```python
from build123d import *

# Parameters (mm, degrees)
SKETCH_1_W          = 106.8
SKETCH_1_H          = 58.8
EXTRUDE_1_DEPTH     = 8
CUT_EXTRUDE_1_DEPTH = 6.08
EXTRUDE_START       = 2.5
EXTRUDE_2_DEPTH     = 2.5
SKETCH_4_W          = 27.87
SKETCH_4_H          = 2.8
CUT_EXTRUDE_2_DEPTH = 4
EXTRUDE_START_2     = 4.5
EXTRUDE_3_DEPTH     = 4.5
SKETCH_6_R          = 1.9
CUT_EXTRUDE_3_DEPTH = 38.5
SKETCH_7_R          = 3.25
CUT_EXTRUDE_4_DEPTH = 3
CHAMFER_7_SIZE      = 0.5
CUT_EXTRUDE_5_DEPTH = 3
CHAMFER_6_SIZE      = 0.5
EXTRUDE_4_DEPTH     = 3
CUT_EXTRUDE_6_DEPTH = 3


with BuildPart() as part:
    # Sketch 1 → Extrude 1 (new body)
    with BuildSketch(Plane(origin=(0, 0, 0), x_dir=(1, 0, 0), z_dir=(0, 1, 0))):
        Rectangle(SKETCH_1_W, SKETCH_1_H)
    extrude(amount=EXTRUDE_1_DEPTH)

    # Sketch 2 → Cut-Extrude 1 (cut)
    with BuildSketch(Plane(origin=(0, 8, 0), x_dir=(1, 0, 0), z_dir=(0, 1, 0))):
        with BuildLine():
            Line((-46.75, -21.5), (46.75, -21.5))
            ThreePointArc((46.75, -21.5), (50.285533906, -20.035533906), (51.75, -16.5))
            Line((51.75, -16.5), (51.75, 24.6))
            ThreePointArc((51.75, 24.6), (51.164213562, 26.014213562), (49.75, 26.6))
            Line((49.75, 26.6), (21.23, 26.6))
            ThreePointArc((21.23, 26.6), (19.815786438, 26.014213562), (19.23, 24.6))
            Line((19.23, 24.6), (19.23, 23.05))
            ThreePointArc((19.23, 23.05), (18.644213562, 21.635786438), (17.23, 21.05))
            Line((17.23, 21.05), (-46.75, 21.05))
            ThreePointArc((-46.75, 21.05), (-50.285533906, 19.585533906), (-51.75, 16.05))
            Line((-51.75, 16.05), (-51.75, -16.5))
            ThreePointArc((-51.75, -16.5), (-50.285533906, -20.035533906), (-46.75, -21.5))
        make_face()
    extrude(amount=-CUT_EXTRUDE_1_DEPTH, mode=Mode.SUBTRACT)

    # Sketch 3 → Extrude 2 (add)
    with BuildSketch(Plane(origin=(0, 8, 0), x_dir=(1, 0, 0), z_dir=(0, 1, 0)).offset(EXTRUDE_START)):
        with BuildLine():
            Line((51.75, 21.1), (53.4, 21.1))
            Line((53.4, 21.1), (53.4, 29.4))
            Line((53.4, 29.4), (49.1, 29.4))
            Line((49.1, 29.4), (49.1, 26.6))
            Line((49.1, 26.6), (49.75, 26.6))
            ThreePointArc((49.75, 26.6), (51.164213562, 26.014213562), (51.75, 24.6))
            Line((51.75, 24.6), (51.75, 21.1))
        make_face()
    extrude(amount=-EXTRUDE_2_DEPTH)

    # Sketch 4 → Cut-Extrude 2 (cut)
    with BuildSketch(Plane(origin=(0, 8, 0), x_dir=(1, 0, 0), z_dir=(0, 1, 0))):
        with Locations((35.165, 28)):
            Rectangle(SKETCH_4_W, SKETCH_4_H)
    extrude(amount=-CUT_EXTRUDE_2_DEPTH, mode=Mode.SUBTRACT)

    # Sketch 5 → Extrude 3 (add)
    with BuildSketch(Plane(origin=(0, 1.92, 0), x_dir=(1, 0, 0), z_dir=(0, 1, 0)).offset(EXTRUDE_START_2)):
        with BuildLine():
            ThreePointArc((-41.983146282, 17.55900816), (-41.590050849, 19.952787734), (-39.42652828, 21.05))
            Line((-39.42652828, 21.05), (-45.440844617, 21.05))
            Line((-45.440844617, 21.05), (-46.75, 21.05))
            ThreePointArc((-46.75, 21.05), (-50.285533906, 19.585533906), (-51.75, 16.05))
            Line((-51.75, 16.05), (-51.75, 8.304033308))
            ThreePointArc((-51.75, 8.304033308), (-50.587117307, 10.675741553), (-48, 11.208770817))
            ThreePointArc((-48, 11.208770817), (-43.12047612, 12.611023931), (-41.983146282, 17.55900816))
        make_face()
        with BuildLine():
            Line((-46.75, -21.5), (-39.004033308, -21.5))
            ThreePointArc((-39.004033308, -21.5), (-41.375741553, -20.337117307), (-41.908770817, -17.75))
            ThreePointArc((-41.908770817, -17.75), (-43.214466094, -12.964466094), (-48, -11.658770817))
            ThreePointArc((-48, -11.658770817), (-50.587117307, -11.125741553), (-51.75, -8.754033308))
            Line((-51.75, -8.754033308), (-51.75, -16.5))
            ThreePointArc((-51.75, -16.5), (-50.285533906, -20.035533906), (-46.75, -21.5))
        make_face()
        with BuildLine():
            Line((51.75, -16.5), (51.75, -8.754033308))
            ThreePointArc((51.75, -8.754033308), (50.587117307, -11.125741553), (48, -11.658770817))
            ThreePointArc((48, -11.658770817), (43.214466094, -12.964466094), (41.908770817, -17.75))
            ThreePointArc((41.908770817, -17.75), (41.375741553, -20.337117307), (39.004033308, -21.5))
            Line((39.004033308, -21.5), (46.75, -21.5))
            ThreePointArc((46.75, -21.5), (50.285533906, -20.035533906), (51.75, -16.5))
        make_face()
        with BuildLine():
            Line((49.75, 19.55), (46.75, 19.55))
            ThreePointArc((46.75, 19.55), (43.25, 16.05), (46.75, 12.55))
            Line((46.75, 12.55), (49.75, 12.55))
            ThreePointArc((49.75, 12.55), (51.164213562, 11.964213562), (51.75, 10.55))
            Line((51.75, 10.55), (51.75, 21.55))
            ThreePointArc((51.75, 21.55), (51.164213562, 20.135786438), (49.75, 19.55))
        make_face()
    extrude(amount=-EXTRUDE_3_DEPTH)

    # Sketch 6 → Cut-Extrude 3 (cut)
    with BuildSketch(Plane(origin=(0, 6.42, 0), x_dir=(1, 0, 0), z_dir=(0, 1, 0))):
        with Locations(Location((-46.75, 16.05, 0), (0, 0, 270))):
            Circle(SKETCH_6_R)
        with Locations(Location((-46.75, -16.5, 0), (0, 0, 270))):
            Circle(SKETCH_6_R)
        with Locations(Location((46.75, -16.5, 0), (0, 0, 270))):
            Circle(SKETCH_6_R)
        with Locations(Location((46.75, 16.05, 0), (0, 0, 270))):
            Circle(SKETCH_6_R)
    extrude(amount=-CUT_EXTRUDE_3_DEPTH, mode=Mode.SUBTRACT)

    # Sketch 7 → Cut-Extrude 4 (cut)
    with BuildSketch(Plane.XZ):
        with Locations(Location((-46.75, 16.5, 0), (0, 0, 270))):
            Circle(SKETCH_7_R)
        with Locations(Location((46.75, 16.5, 0), (0, 0, 270))):
            Circle(SKETCH_7_R)
        with Locations(Location((46.75, -16.05, 0), (0, 0, 270))):
            Circle(SKETCH_7_R)
        with Locations(Location((-46.75, -16.05, 0), (0, 0, 270))):
            Circle(SKETCH_7_R)
    extrude(amount=-CUT_EXTRUDE_4_DEPTH, mode=Mode.SUBTRACT)

    # Chamfer 7
    chamfer_7_edges = [part.edges().sort_by_distance(p)[0] for p in [
        (-46.75, 0, -12.8),
        (46.75, 0, -12.8),
        (46.75, 0, 19.75),
        (-46.75, 0, 19.75),
    ]]
    chamfer(chamfer_7_edges, length=CHAMFER_7_SIZE)

    # Sketch 8 → Cut-Extrude 5 (cut)
    with BuildSketch(Plane(origin=(0, 1.92, 0), x_dir=(1, 0, 0), z_dir=(0, 1, 0))):
        Polygon((17.23, 21.05), (7.83, 21.05), (7.83, -4.95), (33.83, -4.95), (33.83, 21.05), align=None)
    extrude(amount=-CUT_EXTRUDE_5_DEPTH, mode=Mode.SUBTRACT)

    # Chamfer 6
    chamfer_6_edges = [part.edges().sort_by_distance(p)[0] for p in [
        (-53.4, 8, 0),
        (0, 8, 29.4),
        (53.4, 8, 4.15),
        (0, 0, 29.4),
        (49.1, 10.5, -28),
        (49.1, 7.25, -29.4),
        (52.575, 10.5, -21.1),
        (53.4, 9.25, -21.1),
        (-53.4, 0, 0),
        (53.4, 10.5, -25.25),
        (51.25, 10.5, -29.4),
        (0, 0, -29.4),
        (53.4, 0, 0),
        (-16.085, 8, -29.4),
        (35.165, 4, -29.4),
        (21.23, 6, -29.4),
        (21.23, 8, -28),
        (53.4, 4, 29.4),
        (-53.4, 4, 29.4),
        (-53.4, 4, -29.4),
        (53.4, 5.25, -29.4),
    ]]
    chamfer(chamfer_6_edges, length=CHAMFER_6_SIZE)

    # Sketch 11 → Extrude 4 (add)
    with BuildSketch(Plane(origin=(0, 1.92, 0), x_dir=(1, 0, 0), z_dir=(0, 1, 0))):
        Polygon((35.33, -6.45), (35.33, 0.05), (33.83, 0.05), (33.83, -4.95), (28.83, -4.95), (28.83, -6.45), align=None)
        Polygon((6.33, 0.05), (6.33, -6.45), (12.83, -6.45), (12.83, -4.95), (7.83, -4.95), (7.83, 0.05), align=None)
    extrude(amount=EXTRUDE_4_DEPTH)

    # Sketch 12 → Cut-Extrude 6 (cut)
    with BuildSketch(Plane(origin=(0, 1.92, 0), x_dir=(1, 0, 0), z_dir=(0, 1, 0))):
        Polygon((37.922975965, 11.845748795), (36.768275427, 9.845748795), (37.922975965, 7.845748795), (40.232377042, 7.845748795), (41.38707758, 9.845748795), (40.232377042, 11.845748795), align=None)
        Polygon((37.922975965, 6.845748795), (36.768275427, 4.845748795), (37.922975965, 2.845748795), (40.232377042, 2.845748795), (41.38707758, 4.845748795), (40.232377042, 6.845748795), align=None)
        Polygon((42.253102984, 9.345748795), (41.098402446, 7.345748795), (42.253102984, 5.345748795), (44.562504061, 5.345748795), (45.717204599, 7.345748795), (44.562504061, 9.345748795), align=None)
        Polygon((45.717204599, 2.345748795), (44.562504061, 4.345748795), (42.253102984, 4.345748795), (41.098402446, 2.345748795), (42.253102984, 0.345748795), (44.562504061, 0.345748795), align=None)
        Polygon((36.768275427, -0.154251205), (37.922975965, -2.154251205), (40.232377042, -2.154251205), (41.38707758, -0.154251205), (40.232377042, 1.845748795), (37.922975965, 1.845748795), align=None)
    extrude(amount=-CUT_EXTRUDE_6_DEPTH, mode=Mode.SUBTRACT)


solid = part.part
```
Here's how the part is built. I have some questions about the finished solid (model axes, mm). A direction names the side the tool comes from. Round coordinates to 2 decimals unless told otherwise and drop trailing zeros. Loops run counter-clockwise (first coordinate to the right, second up) from the corner with the lowest first, then second, coordinate; pieces in that order, holes last. Notation, with made-up numbers: (23.5, 9.25) -> (42.5, 9.25) arc R7 cw to (42.5, 16.25) -> close; hole circle Ø1 at (15.25, -17). An arc over 180 degrees is marked (long way). Answer as CSV lines item,"result".
1. If I drill on L1, parallel to X at y = 5.4, z = 16.5; L2, parallel to X at y = 2, z = 1.5; L3, parallel to Z at x = 8.5, y = 2, over which ranges is the centre line in solid material (lowest first)?
Final values:
L1,"x = -53.4 to -48.65, -44.85 to -41.75, 41.75 to 44.85, 48.65 to 53.4"
L2,"x = -53.4 to -51.75, 6.33 to 7.83, 33.83 to 35.33, 51.75 to 53.4"
L3,"z = -29.4 to -21.05, 4.95 to 6.45, 21.5 to 29.4"
2. If we section it at A-A on x = -9.5: Please give me the cut outline in (y, z).
Final values:
outline,"(0, -28.9) -> (0.5, -29.4) -> (7.5, -29.4) -> (8, -28.9) -> (8, -21.05) -> (1.92, -21.05) -> (1.92, 21.5) -> (8, 21.5) -> (8, 28.9) -> (7.5, 29.4) -> (0.5, 29.4) -> (0, 28.9) -> close"
3. Thinking about a two-plate mould opening in Z: for faces 1 (the face through (53.4, 4, 0)), 2 (the face through (40.82, 0.97, -5.83)), 3 (the face through (-1, 4, 29.4)), which applies, released by +Z, released by -Z, zero draft, split by the parting line, or undercut?
Final values:
face 1,"zero draft"
face 2,"undercut"
face 3,"released by +Z"
4. Which directions (+Z, -Z, +X, -X, +Y, -Y) give clear straight access to the entire face, cutting with the end or side of a thin tool? Please do faces 4 (the face through (43.25, 4.2, -16.13)), 5 (the face through (21, 1, 4.95)), 6 (the face through (35, 4, -28)).
Final values:
face 4,"+Y"
face 5,"+Y, -Y"
face 6,"-Z, +Y"
5. For pin 1 (3 mm diameter, centred on x = 16, z = 16, fed in from +Y); pin 2 (3 mm diameter, centred on x = 33.5, z = 3, fed in from +Y); pin 3 (4 mm diameter, centred on x = 8.5, z = -20, fed in from +Y), each with a flat end and sliding along its axis, tell me the tip position at first contact or that it passes through.
Final values:
pin 1,"stops at y = 1.92"
pin 2,"stops at y = 4.92"
pin 3,"stops at y = 8"
